Here's how the part is built. I have some questions about the finished solid (model axes, mm). Round coordinates to 2 decimals unless told otherwise and drop trailing zeros. Write each loop counter-clockwise with the first axis right and the second up, starting at its lowest first coordinate (ties: lowest second). Pieces come first, ordered by that corner, then holes. Notation, with made-up numbers: (42.5, 38.25) -> (86.5, 38.25) arc R20 ccw to (86.5, 64.25) -> close; hole circle Ø5 at (-14.5, -9.5). An arc over 180 degrees is marked (long way). Answer in a Markdown table with one row per item.
from build123d import *

# Parameters (mm, degrees)
CROQUIS1_R                       = 2.5
SALIENTE_EXTRUIR1_DEPTH          = 1.5875
TALADRO_DE_MARGEN_PARA_M31_D     = 3.4
TALADRO_DE_MARGEN_PARA_M31_DEPTH = 10
TALADRO_DE_MARGEN_PARA_M31_TIP   = 1.021463052


with BuildPart() as part:
    # Croquis1 → Saliente-Extruir1 (new, symmetric)
    with BuildSketch(Plane(origin=(0, 0, 0), x_dir=(1, 0, 0), z_dir=(0, 1, 0))):
        with BuildLine():
            Line((52, 40), (-52, 40))
            ThreePointArc((-52, 40), (-54.121320344, 39.121320344), (-55, 37))
            Line((-55, 37), (-55, -37))
            ThreePointArc((-55, -37), (-54.121320344, -39.121320344), (-52, -40))
            Line((-52, -40), (52, -40))
            ThreePointArc((52, -40), (54.121320344, -39.121320344), (55, -37))
            Line((55, -37), (55, 37))
            ThreePointArc((55, 37), (54.121320344, 39.121320344), (52, 40))
        make_face()
        with Locations(Location((34.5, 30, 0), (0, 0, 270))):
            Circle(CROQUIS1_R, mode=Mode.SUBTRACT)
        with Locations(Location((34.5, -30, 0), (0, 0, 270))):
            Circle(CROQUIS1_R, mode=Mode.SUBTRACT)
        with Locations(Location((-34.5, -30, 0), (0, 0, 270))):
            Circle(CROQUIS1_R, mode=Mode.SUBTRACT)
        with Locations(Location((-34.5, 30, 0), (0, 0, 270))):
            Circle(CROQUIS1_R, mode=Mode.SUBTRACT)
    extrude(amount=SALIENTE_EXTRUIR1_DEPTH, both=True)

    # Taladro de margen para M31
    with Locations(Plane(origin=(0, 1.5875, 0), x_dir=(1, 0, 0), z_dir=(0, 1, 0))):
        with Locations((0, 13), (12.363734712, 4.017220927), (7.64120828, -10.517220927), (-7.64120828, -10.517220927), (-12.363734712, 4.017220927)):
            Hole(TALADRO_DE_MARGEN_PARA_M31_D / 2, depth=TALADRO_DE_MARGEN_PARA_M31_DEPTH)
            with Locations((0, 0, -(TALADRO_DE_MARGEN_PARA_M31_DEPTH + TALADRO_DE_MARGEN_PARA_M31_TIP / 2))):  # 118° drill point
                Cone(0, TALADRO_DE_MARGEN_PARA_M31_D / 2, TALADRO_DE_MARGEN_PARA_M31_TIP, mode=Mode.SUBTRACT)


solid = part.part
1) I want a section at B-B, the plane z = -30. List the corners of the cut face in (x, y) for me, and give its area (4 significant figures).
Response:
| item | result |
|---|---|
| outline | (-55, -1.59) -> (-37, -1.59) -> (-37, 1.59) -> (-55, 1.59) -> close; (-32, -1.59) -> (32, -1.59) -> (32, 1.59) -> (-32, 1.59) -> close; (37, -1.59) -> (55, -1.59) -> (55, 1.59) -> (37, 1.59) -> close |
| area | 317.5 mm^2 |
2) I want a section at C-C, the plane x = -34.5. List the corners of the cut face in (y, z) for me.
Response:
| item | result |
|---|---|
| outline | (-1.59, -40) -> (1.59, -40) -> (1.59, -32.5) -> (-1.59, -32.5) -> close; (-1.59, -27.5) -> (1.59, -27.5) -> (1.59, 27.5) -> (-1.59, 27.5) -> close; (-1.59, 32.5) -> (1.59, 32.5) -> (1.59, 40) -> (-1.59, 40) -> close |
3) I want a section at D-D, the plane x = 0. List the corners of the cut face in (y, z) for me, and give its area (3 significant figures).
Response:
| item | result |
|---|---|
| outline | (-1.59, -40) -> (1.59, -40) -> (1.59, -14.7) -> (-1.59, -14.7) -> close; (-1.59, -11.3) -> (1.59, -11.3) -> (1.59, 40) -> (-1.59, 40) -> close |
| area | 243 mm^2 |
4) I want a section at A-A, the plane z = -13. List the corners of the cut face in (x, y) for me, and give its area (3 significant figures).
Response:
| item | result |
|---|---|
| outline | (-55, -1.59) -> (-1.7, -1.59) -> (-1.7, 1.59) -> (-55, 1.59) -> close; (1.7, -1.59) -> (55, -1.59) -> (55, 1.59) -> (1.7, 1.59) -> close |
| area | 338 mm^2 |
5) I need wall thicknesses on line 1 (X direction, y = -0.6, z = -30); line 2 (Z direction, x = 0, y = 0.05); line 3 (X direction, y = -1.25, z = -30.5). Which ranges of each line are inside material? Lowest first, please. Write a range as [from, to].
Response:
| item | result |
|---|---|
| line 1 | x = [-55, -37], [-32, 32], [37, 55] |
| line 2 | z = [-40, -14.7], [-11.3, 40] |
| line 3 | x = [-55, -36.95], [-32.05, 32.05], [36.95, 55] |
6) For pin 1 (2 mm diameter, centred on x = 12.36, z = -4.02, fed in from -Y), with a flat end and sliding along its axis, tell me the tip position at first contact or that it passes through.
Response:
| item | result |
|---|---|
| pin 1 | passes through |
7) We'd pull the mould along Z, two halves only. Please class faces 1 (the face through (-54.14, 0.02, 39.1)), 2 (the face through (-1, -1.588, -1)), 3 (the face through (7.86, -0.02, 8.83)): +Z half, -Z half, draft (parallel to the pull), parting line (faces both ways), or undercut.
Response:
| item | result |
|---|---|
| face 1 | +Z half |
| face 2 | draft |
| face 3 | undercut |
